```python
from build123d import *

# Parameters (mm, degrees)
BOSS_EXTRUDE1_DEPTH = 5
SKETCH2_R           = 7.25
BOSS_EXTRUDE2_DEPTH = 5
SKETCH5_R           = 6
CUT_EXTRUDE2_DEPTH  = 1
SKETCH6_R           = 2
CUT_EXTRUDE3_DEPTH  = 4
FILLET1_R           = 3
SKETCH7_R           = 5.25
CUT_EXTRUDE4_DEPTH  = 3


with BuildPart() as part:
    # Sketch1 → Boss-Extrude1 (new body)
    with BuildSketch(Plane.XY):
        with BuildLine():
            Line((-68.758315939, 4), (-12.748315939, 4))
            ThreePointArc((-12.748315939, 4), (-8.748315939, 0), (-12.748315939, -4))
            Line((-12.748315939, -4), (-68.758315939, -4))
            ThreePointArc((-68.758315939, -4), (-72.758315939, 0), (-68.758315939, 4))
        make_face()
    extrude(amount=BOSS_EXTRUDE1_DEPTH)

    # Sketch2 → Boss-Extrude2 (add)
    with BuildSketch(Plane(origin=(0, 0, 0), x_dir=(-1, 0, 0), z_dir=(0, 0, -1))):
        with Locations((40.753315939, 0)):
            Circle(SKETCH2_R)
        with Locations((68.758315939, 0)):
            Circle(SKETCH2_R)
        with Locations((12.748315939, 0)):
            Circle(SKETCH2_R)
    extrude(amount=-BOSS_EXTRUDE2_DEPTH)

    # Sketch5 → Cut-Extrude2 (cut)
    with BuildSketch(Plane.XY.offset(5)):
        with Locations((-68.758315939, 0)):
            Circle(SKETCH5_R)
        with Locations((-40.753315939, 0)):
            Circle(SKETCH5_R)
        with Locations((-12.748315939, 0)):
            Circle(SKETCH5_R)
    extrude(amount=-CUT_EXTRUDE2_DEPTH, mode=Mode.SUBTRACT)

    # Sketch6 → Cut-Extrude3 (cut)
    with BuildSketch(Plane(origin=(0, 0, 0), x_dir=(-1, 0, 0), z_dir=(0, 0, -1))):
        with Locations((12.748315939, 0)):
            Circle(SKETCH6_R)
        with Locations((40.753315939, 0)):
            Circle(SKETCH6_R)
        with Locations(Location((68.758315939, 0, 0), (0, 0, 180))):
            Circle(SKETCH6_R)
    extrude(amount=-CUT_EXTRUDE3_DEPTH, mode=Mode.SUBTRACT)

    # Fillet1
    fillet1_edges = [part.edges().sort_by_distance(p)[0] for p in [
        (-34.706622628, -4, 2.5),
        (-34.706622628, 4, 2.5),
        (-46.80000925, -4, 2.5),
        (-46.80000925, 4, 2.5),
        (-62.711622628, 4, 2.5),
        (-62.711622628, -4, 2.5),
        (-18.79500925, -4, 2.5),
        (-18.79500925, 4, 2.5),
    ]]
    fillet(fillet1_edges, radius=FILLET1_R)

    # Sketch7 → Cut-Extrude4 (cut)
    with BuildSketch(Plane.XY.offset(4)):
        with Locations((-68.758315939, 0)):
            Circle(SKETCH7_R)
        with Locations((-40.753315939, 0)):
            Circle(SKETCH7_R)
        with Locations((-12.748315939, 0)):
            Circle(SKETCH7_R)
    extrude(amount=-CUT_EXTRUDE4_DEPTH, mode=Mode.SUBTRACT)


solid = part.part
```
The model under review builds one solid part; all positions refer to its coordinate system, in mm. A direction names the side the tool comes from. Give positions to 0.01 mm unless a question says otherwise; leave off trailing zeros. Write each loop counter-clockwise with the first axis right and the second up, starting at its lowest first coordinate (ties: lowest second). Pieces come first, ordered by that corner, then holes.
(1) Consider section D-D, the plane x = -34. Give the boundary of the cut face in (y, z).
(2) For P1, Ø3, axis at x = -41.5, y = -1.5, coming from the +Z side; P2, Ø2.5, axis at x = -23.5, z = 2, coming from the +Y side; P3, Ø6, axis at x = -13.5, y = -2.5, coming from the +Z side; P4, Ø2.5, axis at x = -12.75, y = 0, coming from the -Z side, all flat-tipped, find the tip position at first contact; note any pin that passes through.
(3) Consider section B-B, the plane x = -55. Give the boundary of the cut face in (y, z).
(4) Consider section C-C, the plane y = 0. Give the number of separate pieces and of enclosed holes in the cut face, and give its area (3 significant figures).
(5) To check wall thickness, follow L1, parallel to X at y = -0.5, z = 4.5; L2, parallel to X at y = 1.25, z = 4.85; L3, parallel to X at y = -4.25, z = 0.7. State the ranges of each line that lie inside material, in increasing order.
(6) Consider section A-A, the plane z = 2.5. Give the boundary of the cut face in (x, y), and give its area (3 significant figures).
(7) Tool access review of faces 1 (the cylindrical face through (-19.026, 4.255, 2.465)), 2 (the cylindrical face through (-46, 0.2, 2.5)), 3 (the flat face through (-55, -4, 2)): name each direction out of +Z, -Z, +X, -X, +Y, -Y from which nothing blocks a thin tool from reaching the whole face with its end or side.
Returned:
1. outline: (-4.09, 0) - (4.09, 0) - (4.09, 5) - (-4.09, 5) - close
2. P1: stops at z = 1
2. P2: stops at y = 4
2. P3: stops at z = 4
2. P4: passes through
3. outline: (-4, 0) - (4, 0) - (4, 5) - (-4, 5) - close
4. separate pieces: 4
4. enclosed holes: 0
4. area: 210 mm2
5. L1: x = -75.99 to -74.74, -62.78 to -46.73, -34.77 to -18.73, -6.77 to -5.52
5. L2: x = -75.9 to -74.63, -62.89 to -46.62, -34.88 to -18.62, -6.88 to -5.61
5. L3: x = -74.63 to -62.47, -47.04 to -34.46, -19.04 to -6.87
6. outline: (-63.46, -4.95) arc R3 cw to (-61.27, -4) - (-48.24, -4) arc R3 cw to (-46.05, -4.95) arc R7.25 ccw to (-35.46, -4.95) arc R3 cw to (-33.27, -4) - (-20.24, -4) arc R3 cw to (-18.04, -4.95) arc R7.25 ccw (long way) to (-18.04, 4.95) arc R3 cw to (-20.24, 4) - (-33.27, 4) arc R3 cw to (-35.46, 4.95) arc R7.25 ccw to (-46.05, 4.95) arc R3 cw to (-48.24, 4) - (-61.27, 4) arc R3 cw to (-63.46, 4.95) arc R7.25 ccw (long way) to start; hole circle Ø10.5 at (-68.76, 0); hole circle Ø10.5 at (-40.75, 0); hole circle Ø10.5 at (-12.75, 0)
6. area: 466 mm2
7. face 1: +Z, -Z, +Y
7. face 2: +Z
7. face 3: +Z, -Z, -Y
